Geometry: final body of the model. Coordinates: model frame, mm. Coordinates: 2 decimals unless noted, no trailing zeros. Order: outer loops, then holes, each group sorted by start corner. A loop starts at its lowest first (then second) coordinate and runs counter-clockwise, first axis right, second up. Notation, with made-up numbers: M 73,-11 L 114,-11 A13 cw 114,5 Z; hole C -16,89 d11. An arc over 180 degrees is marked long. Use CSV: the item, a comma, the result in double quotes. Start each with the question number.
Q1. Ray query, probe 1 along X at (y, z) = (5, 0.85); probe 2 along Z at (x, y) = (7.75, 6); probe 3 along Z at (x, y) = (10, 3.75). Return the intervals inside material, ascending.
Q2. Section query A-A, the plane x = 5. Output: boundary loops of the cut face in (y, z).
Q3. Section query C-C, the plane z = 5. Output: boundary loops of the cut face in (x, y).
Q4. Section query B-B, the plane x = 2.75. Output: boundary loops of the cut face in (y, z), and give its area (3 significant figures).
Q5. Section query D-D, the plane y = 5. Output: boundary loops of the cut face in (x, z), and give its area (3 significant figures).
Q6. Mould query, pull axis Z, two halves, no side actions, for faces 1 (the face through (13.56, 5.98, 1.9)), 2 (the face through (9, 10, 5)), 3 (the face through (4.44, 3.85, 7.77)), 4 (the face through (9, 5, 10)). Classes: +Z half, -Z half, draft (parallel to the pull), parting line (faces both ways), or undercut.
from build123d import *

# Parameters (mm, degrees)
SKETCH_1_W          = 10
SKETCH_1_H          = 10
EXTRUDE_2_DEPTH     = 18
SKETCH_2_R          = 3.25
CUT_EXTRUDE_1_DEPTH = 9
SKETCH_3_R          = 3
CUT_EXTRUDE_2_DEPTH = 15
SKETCH_4_R          = 1
CUT_EXTRUDE_3_DEPTH = 10
FILLET_1_R          = 2


with BuildPart() as part:
    # 草图1 → 凸台-拉伸2 (new body)
    with BuildSketch(Plane(origin=(0, 0, 0), x_dir=(0, 0, -1), z_dir=(1, 0, 0))):
        with Locations((-5, 5)):
            Rectangle(SKETCH_1_W, SKETCH_1_H)
    extrude(amount=EXTRUDE_2_DEPTH)

    # 草图2 → 切除-拉伸1 (cut)
    with BuildSketch(Plane(origin=(18, 0, 0), x_dir=(0, 0, -1), z_dir=(1, 0, 0))):
        with Locations((-5, 5)):
            Circle(SKETCH_2_R)
    extrude(amount=-CUT_EXTRUDE_1_DEPTH, mode=Mode.SUBTRACT)

    # 草图3 → 切除-拉伸2 (cut)
    with BuildSketch(Plane.ZY):
        with Locations((5, 5)):
            Circle(SKETCH_3_R)
    extrude(amount=-CUT_EXTRUDE_2_DEPTH, mode=Mode.SUBTRACT)

    # 草图4 → 切除-拉伸3 (cut)
    with BuildSketch(Plane(origin=(0, 0, 0), x_dir=(-1, 0, 0), z_dir=(0, 0, -1))):
        with Locations(Location((-15, 5, 0), (0, 0, 90))):
            Circle(SKETCH_4_R)
        with Locations(Location((-5, 5, 0), (0, 0, 90))):
            Circle(SKETCH_4_R)
    extrude(amount=-CUT_EXTRUDE_3_DEPTH, mode=Mode.SUBTRACT)

    # 圆角1
    fillet_1_edges = [part.edges().sort_by_distance(p)[0] for p in [
        (9, 0, 0),
        (9, 10, 0),
        (9, 10, 10),
        (9, 0, 10),
    ]]
    fillet(fillet_1_edges, radius=FILLET_1_R)


solid = part.part
Responses:
1,probe 1,"x = 0 to 4, 6 to 14, 16 to 18"
1,probe 2,"z = 0 to 2.17, 7.83 to 10"
1,probe 3,"z = 0 to 2, 8 to 10"
2,outline,"M 0,2 A2 ccw 2,0 L 4,0 L 4,2.17 A3 cw 4,7.83 L 4,10 L 2,10 A2 ccw 0,8 Z; M 6,0 L 8,0 A2 ccw 10,2 L 10,8 A2 ccw 8,10 L 6,10 L 6,7.83 A3 cw 6,2.17 Z"
3,outline,"M 0,0 L 18,0 L 18,1.75 L 9,1.75 L 9,2 L 0,2 Z; M 0,8 L 9,8 L 9,8.25 L 18,8.25 L 18,10 L 0,10 Z"
4,outline,"M 0,2 A2 ccw 2,0 L 8,0 A2 ccw 10,2 L 10,8 A2 ccw 8,10 L 2,10 A2 ccw 0,8 Z; hole C 5,5 d6"
4,area,"68.3 mm²"
5,outline,"M 0,0 L 4,0 L 4,2 L 0,2 Z; M 0,8 L 4,8 L 4,10 L 0,10 Z; M 6,0 L 14,0 L 14,1.75 L 9,1.75 L 9,2 L 6,2 Z; M 6,8 L 9,8 L 9,8.25 L 14,8.25 L 14,10 L 6,10 Z; M 16,0 L 18,0 L 18,1.75 L 16,1.75 Z; M 16,8.25 L 18,8.25 L 18,10 L 16,10 Z"
5,area,"52.5 mm²"
6,face 1,"undercut"
6,face 2,"draft"
6,face 3,"undercut"
6,face 4,"+Z half"
